Here's how the part is built. I have some questions about the finished solid (model axes, mm). Face numbers are marked on the shaded views. A direction names the side the tool comes from. Round coordinates to 2 decimals unless told otherwise and drop trailing zeros. Write each loop counter-clockwise with the first axis right and the second up, starting at its lowest first coordinate (ties: lowest second). Pieces come first, ordered by that corner, then holes. Notation, with made-up numbers: (39, 0.5) -> (85, 0.5) arc R20 ccw to (85, 7.5) -> close; hole circle Ø8 at (-4, 4). An arc over 180 degrees is marked (long way). Answer as CSV lines item,"result".
```python
from build123d import *

# Parameters (mm, degrees)
BOSS_EXTRUDE2_DEPTH     = 2.5
SKETCH2_R               = 5
BOSS_EXTRUDE3_DEPTH     = 3
LPATTERN1_COUNT         = 2
LPATTERN1_PITCH         = 53
MIRROR8_COPY_1_SKETCH_R = 5
MIRROR8_COPY_1_DEPTH    = 3
SKETCH4_W               = 30
SKETCH4_H               = 2.5
BOSS_EXTRUDE4_DEPTH     = 35
SKETCH6_R               = 3.75
SKETCH6_R_2             = 1.5
CUT_EXTRUDE1_DEPTH      = 2.5


with BuildPart() as part:
    # Sketch1 → Boss-Extrude2 (new body)
    with BuildSketch(Plane.XY):
        with BuildLine():
            Line((-120, 0), (-61.0553028, 0))
            ThreePointArc((-61.0553028, 0), (-48.351787131, -0.674308342), (-35.791039572, -2.689655172))
            ThreePointArc((-35.791039572, -2.689655172), (0, -6.5), (35.791039572, -2.689655172))
            ThreePointArc((35.791039572, -2.689655172), (48.351787131, -0.674308342), (61.0553028, 0))
            Line((61.0553028, 0), (120, 0))
            Line((120, 0), (120, 20))
            Line((120, 20), (56.637002039, 20))
            ThreePointArc((56.637002039, 20), (45.235247788, 19.347873656), (33.982201224, 17.4))
            ThreePointArc((33.982201224, 17.4), (0, 13.5), (-33.982201224, 17.4))
            ThreePointArc((-33.982201224, 17.4), (-45.235247788, 19.347873656), (-56.637002039, 20))
            Line((-56.637002039, 20), (-120, 20))
            Line((-120, 20), (-120, 0))
        make_face()
    extrude(amount=BOSS_EXTRUDE2_DEPTH)


with BuildPart() as body_2:
    # Mirror7: mirrored copy
    add(part.part.mirror(Plane.XY.offset(-15)))


with BuildPart() as part_1:
    add(part.part)

    add(body_2.part)  # Boss-Extrude3 merges body 2
    # Sketch2 → Boss-Extrude3 (add)
    with BuildSketch(Plane(origin=(120, 0, 0), x_dir=(0, 0, -1), z_dir=(1, 0, 0))):
        with BuildLine():
            Line((0, 20), (0, 0))
            ThreePointArc((0, 0), (15, -8.027756377), (30, 0))
            Line((30, 0), (30, 20))
            ThreePointArc((30, 20), (15, 28.027756377), (0, 20))
        make_face()
        with Locations((15, 10)):
            Circle(SKETCH2_R, mode=Mode.SUBTRACT)
    boss_extrude3 = extrude(amount=-BOSS_EXTRUDE3_DEPTH)

    # LPattern1: Boss-Extrude3 ×2
    with Locations(*[(-i * LPATTERN1_PITCH, 0, 0) for i in range(1, LPATTERN1_COUNT)]):
        add(boss_extrude3)

    # Mirror8: Boss-Extrude3 across plane
    add(boss_extrude3.mirror(Plane(origin=(0, 0, 0), x_dir=(0, 0, 1), z_dir=(1, 0, 0))))

    # Mirror8 copy 1 sketch → Mirror8 copy 1 (add)
    with BuildSketch(Plane(origin=(-67, 0, 0), x_dir=(0, 0, -1), z_dir=(-1, 0, 0))):
        with BuildLine():
            Line((0, -20), (0, 0))
            ThreePointArc((0, 0), (15, 8.027756377), (30, 0))
            Line((30, 0), (30, -20))
            ThreePointArc((30, -20), (15, -28.027756377), (0, -20))
        make_face()
        with Locations((15, -10)):
            Circle(MIRROR8_COPY_1_SKETCH_R, mode=Mode.SUBTRACT)
    extrude(amount=-MIRROR8_COPY_1_DEPTH)

    # Sketch4 → Boss-Extrude4 (add)
    with BuildSketch(Plane(origin=(0, 0, -32.5), x_dir=(-1, 0, 0), z_dir=(0, 0, -1))):
        with Locations((0, 12.25)):
            Rectangle(SKETCH4_W, SKETCH4_H)
    extrude(amount=-BOSS_EXTRUDE4_DEPTH)

    # Sketch6 → Cut-Extrude1 (cut)
    with BuildSketch(Plane(origin=(0, 13.5, 0), x_dir=(1, 0, 0), z_dir=(0, 1, 0))):
        with Locations((0, 15)):
            Circle(SKETCH6_R)
        with Locations((-7.5, 22.5)):
            Circle(SKETCH6_R_2)
        with Locations((7.5, 22.5)):
            Circle(SKETCH6_R_2)
        with Locations((7.5, 7.5)):
            Circle(SKETCH6_R_2)
        with Locations((-7.5, 7.5)):
            Circle(SKETCH6_R_2)
    extrude(amount=-CUT_EXTRUDE1_DEPTH, mode=Mode.SUBTRACT)


solid = part_1.part
```
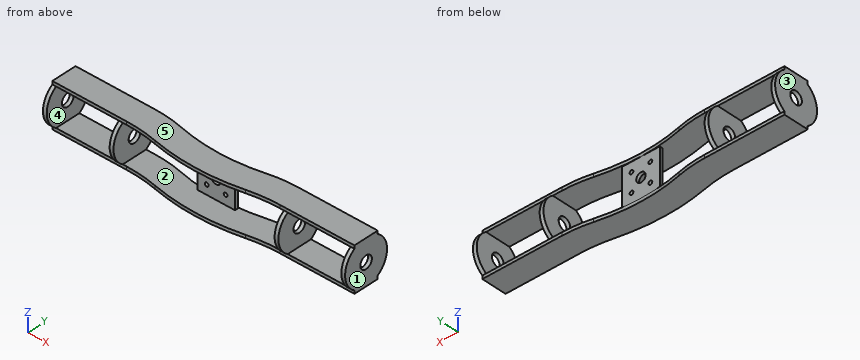
1. On a 3-axis mill with a long thin cutter (end or side, diameter ignored), from which of +Z, -Z, +X, -X, +Y, -Y can I reach the whole of each face in a straight line? I mean the marked faces 4 and 5. Say none if no direction works.
Numbers:
face 4,"+Y, -Y"
face 5,"+Z, +X, -X, +Y, -Y"
2. For pin 1 Ø3 at (x, z) = (97.5, -31.5) entering from +Y; pin 2 Ø6 at (x, z) = (10, -19) entering from -Y; pin 3 Ø3 at (x, z) = (97, -31.5) entering from -Y; pin 4 Ø11.5 at (y, z) = (10, -15) entering from -X, each with a flat end and sliding along its axis, tell me the tip position at first contact or that it passes through.
Numbers:
pin 1,"stops at y = 20"
pin 2,"stops at y = 11"
pin 3,"stops at y = 0"
pin 4,"stops at x = -120"
3. If I drill on line 1 (X direction, y = 22.5, z = -15); line 2 (Z direction, x = 38, y = 11.5); line 3 (Z direction, x = 0, y = 11.75), over which ranges is the centre line in solid material (lowest first)?
Numbers:
line 1,"x = -120 to -117, -67 to -64, 64 to 67, 117 to 120"
line 2,"z = -32.5 to -30, 0 to 2.5"
line 3,"z = -32.5 to -18.75, -11.25 to 2.5"
4. Suppose I cut it at A-A on x = 88.5. Please give me the cut outline in (y, z), and give its area (3 significant figures).
Numbers:
outline,"(0, -32.5) -> (20, -32.5) -> (20, -30) -> (0, -30) -> close; (0, 0) -> (20, 0) -> (20, 2.5) -> (0, 2.5) -> close"
area,"100 mm^2"
5. If we mould it in two halves opening along X, with no side actions, what happens to the marked faces 1, 2 and 3? For each: released by +X, released by -X, zero draft, split by the parting line, or undercut.
Numbers:
face 1,"released by +X"
face 2,"undercut"
face 3,"released by -X"
